from build123d import *

# Parameters (mm, degrees)
F0_W     = 381
F0_H     = 254
F0_W_2   = 127
F0_H_2   = 88.9
F1_DEPTH = 10.16
F2_W     = 127
F2_H     = 88.9
F3_DEPTH = 38.1
F4_W     = 116.84
F4_H     = 78.74
F5_DEPTH = 20.32


with BuildPart() as f1:
    # F0 (on Top) → F1 (new body)
    with BuildSketch(Plane.XY):
        with Locations((0.95677, 23.492131)):
            Rectangle(F0_W, F0_H)
        with Locations((-87.94323, -44.45)):
            Rectangle(F0_W_2, F0_H_2, mode=Mode.SUBTRACT)
        with Locations((89.85677, -44.593953)):
            Rectangle(F0_W_2, F0_H_2, mode=Mode.SUBTRACT)
        with Locations((-87.94323, -44.45)):
            Rectangle(F0_W_2, F0_H_2)
        with Locations((89.85677, -44.593953)):
            Rectangle(F0_W_2, F0_H_2)
    extrude(amount=F1_DEPTH)

    # F2 (on face) → F3 (join)
    with BuildSketch(Plane.XY.offset(10.16)):
        with Locations((-87.94323, 80.642131)):
            Rectangle(F2_W, F2_H)
        with Locations((89.85677, 80.642131)):
            Rectangle(F2_W, F2_H)
    extrude(amount=-F3_DEPTH)

    # F4 (on face) → F5 (cut)
    with BuildSketch(Plane.XY.offset(10.16)):
        with Locations((-87.94323, 80.642131)):
            Rectangle(F4_W, F4_H)
        with Locations((89.85677, 80.642131)):
            Rectangle(F4_W, F4_H)
    extrude(amount=-F5_DEPTH, mode=Mode.SUBTRACT)


solid = f1.part
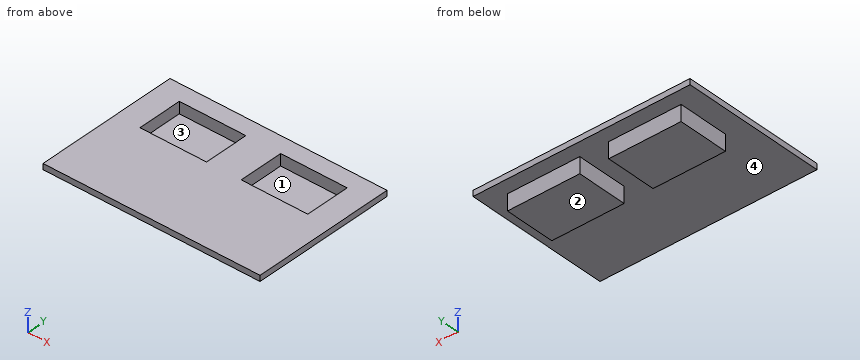
Build history of the part. All positions in model axes, mm. Face numbers are marked on the shaded views. A direction names the side the tool comes from. Round coordinates to 2 decimals unless told otherwise and drop trailing zeros. Write each loop counter-clockwise with the first axis right and the second up, starting at its lowest first coordinate (ties: lowest second). Pieces come first, ordered by that corner, then holes. Notation, with made-up numbers: M 50,57.5 L 84,57.5 A18 cw 84,81.5 Z; hole C 28.5,1 d2. An arc over 180 degrees is marked long. Use CSV: the item, a comma, the result in double quotes.
1. Saw through at C-C (x = 65.5). Give the cut face in (y, z).
Reply:
outline,"M -103.51,0 L 36.19,0 L 36.19,-27.94 L 125.09,-27.94 L 125.09,0 L 150.49,0 L 150.49,10.16 L 120.01,10.16 L 120.01,-10.16 L 41.27,-10.16 L 41.27,10.16 L -103.51,10.16 Z"
2. Two-plate mould, pull along Y, no slides. Class the marked faces 3 and 4: +Y half, -Y half, draft (parallel to the pull), parting line (faces both ways), or undercut.
Reply:
face 3,"undercut"
face 4,"draft"
3. Wall check: probe 1 along X at (y, z) = (63, -6); probe 2 along Y at (x, z) = (63.5, 7.5); probe 3 along X at (y, z) = (41.5, -16). Give the ranges that are in metal, low to high. Write a range as from..to.
Reply:
probe 1,"x = -151.44..-146.36, -29.52..-24.44, 26.36..31.44, 148.28..153.36"
probe 2,"y = -103.51..41.27, 120.01..150.49"
probe 3,"x = -151.44..-24.44, 26.36..153.36"
4. Saw through at B-B (z = 5). Give the cut face in (x, y), plus the area to 3 significant figures.
Reply:
outline,"M -189.54,-103.51 L 191.46,-103.51 L 191.46,150.49 L -189.54,150.49 Z; hole M -146.36,41.27 L -29.52,41.27 L -29.52,120.01 L -146.36,120.01 Z; hole M 31.44,41.27 L 148.28,41.27 L 148.28,120.01 L 31.44,120.01 Z"
area,"78,400 mm²"
5. Saw through at A-A (z = -16). Give the cut face in (x, y), plus the area to 3 significant figures.
Reply:
outline,"M -151.44,36.19 L -24.44,36.19 L -24.44,125.09 L -151.44,125.09 Z; M 26.36,36.19 L 153.36,36.19 L 153.36,125.09 L 26.36,125.09 Z"
area,"22,600 mm²"
6. Saw through at D-D (y = 68). Give the cut face in (x, z).
Reply:
outline,"M -189.54,0 L -151.44,0 L -151.44,-27.94 L -24.44,-27.94 L -24.44,0 L 26.36,0 L 26.36,-27.94 L 153.36,-27.94 L 153.36,0 L 191.46,0 L 191.46,10.16 L 148.28,10.16 L 148.28,-10.16 L 31.44,-10.16 L 31.44,10.16 L -29.52,10.16 L -29.52,-10.16 L -146.36,-10.16 L -146.36,10.16 L -189.54,10.16 Z"
7. Tool access for the marked faces 1 and 2: list every direction of +Z, -Z, +X, -X, +Y, -Y with a clear straight run to the whole face (end or side of a thin tool).
Reply:
face 1,"+Z"
face 2,"-Z, +X, -X, +Y, -Y"
8. Flat gauge pins, fed straight in: pin 1 (6 mm diameter, centred on x = -77.5, y = 86, fed in from +Z); pin 2 (8 mm diameter, centred on x = 151.5, z = -13.5, fed in from -Y); pin 3 (10 mm diameter, centred on x = 88, y = 29.5, fed in from -Z). Where does each tip first touch, or does it go through?
Reply:
pin 1,"stops at z = -10.16"
pin 2,"stops at y = 36.19"
pin 3,"stops at z = 0"
